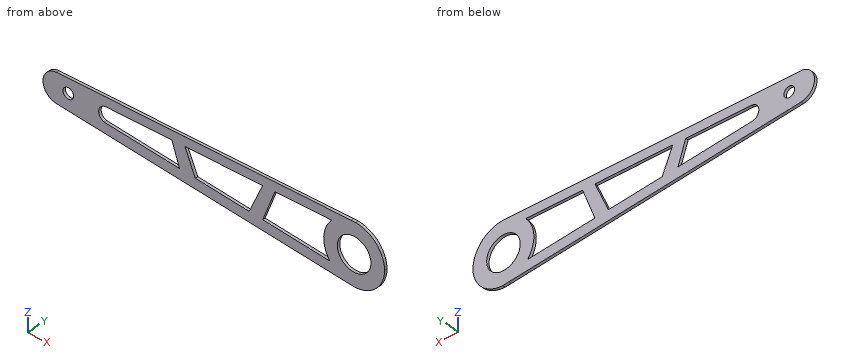
from build123d import *

# Parameters (mm, degrees)
F1_DEPTH = 0.739
F2_R     = 4.5593
F3_DEPTH = 25.4
F4_R     = 1.447766
F5_DEPTH = 25.4


with BuildPart() as f1:
    # F0 (on Front) → F1 (new body)
    with BuildSketch(Plane.XZ):
        with BuildLine():
            ThreePointArc((27.782233, 3.263093), (30.16178, 5.045361), (33.017843, 5.870969))
            Line((33.017843, 5.870969), (-46.981648, 3.796947))
            ThreePointArc((-46.981648, 3.796947), (-50.678208, -0.180343), (-46.9984, -4.173137))
            Line((-46.9984, -4.173137), (32.345508, -10.48937))
            ThreePointArc((32.345508, -10.48937), (29.496427, -9.389113), (27.240975, -7.329802))
            Line((27.240975, -7.329802), (9.005115, -5.878122))
            Line((9.005115, -5.878122), (5.326605, -5.585291))
            Line((5.326605, -5.585291), (-9.280345, -4.422494))
            Line((-9.280345, -4.422494), (-13.580459, -4.08018))
            Line((-13.580459, -4.08018), (-34.080148, -2.448286))
            ThreePointArc((-34.080148, -2.448286), (-35.521395, -0.140366), (-33.488405, 1.668126))
            Line((-33.488405, 1.668126), (-15.681088, 2.131677))
            Line((-15.681088, 2.131677), (-12.137563, 2.223921))
            Line((-12.137563, 2.223921), (9.005115, 2.774297))
            Line((9.005115, 2.774297), (12.333791, 2.860947))
            Line((12.333791, 2.860947), (27.782233, 3.263093))
        make_face()
        with BuildLine():
            ThreePointArc((34.046986, -10.624817), (39.766374, -8.134536), (42.119023, -2.357172))
            ThreePointArc((42.119023, -2.357172), (39.837821, 3.346097), (34.252707, 5.902984))
            Line((34.252707, 5.902984), (33.017843, 5.870969))
            ThreePointArc((33.017843, 5.870969), (30.16178, 5.045361), (27.782233, 3.263093))
            ThreePointArc((27.782233, 3.263093), (25.589768, -1.935156), (27.240975, -7.329802))
            ThreePointArc((27.240975, -7.329802), (29.496427, -9.389113), (32.345508, -10.48937))
            Line((32.345508, -10.48937), (34.046986, -10.624817))
        make_face()
        Polygon((9.005115, -5.878122), (12.333791, 2.860947), (9.005115, 2.774297), (5.326605, -5.585291), align=None)
        Polygon((-9.280345, -4.422494), (-12.137563, 2.223921), (-15.681088, 2.131677), (-13.580459, -4.08018), align=None)
    extrude(amount=F1_DEPTH)

    # F2 (on face) → F3 (cut)
    with BuildSketch(Plane.XZ.offset(0.739)):
        with Locations((33.849008, -2.357172)):
            Circle(F2_R)
    extrude(amount=-F3_DEPTH, mode=Mode.SUBTRACT)

    # F4 (on face) → F5 (cut)
    with BuildSketch(Plane.XZ.offset(0.739)):
        with Locations((-43.807384, 0)):
            Circle(F4_R)
    extrude(amount=-F5_DEPTH, mode=Mode.SUBTRACT)


solid = f1.part
Can you work these out from the model? Positions are in its coordinate system, mm. Coordinates: 2 decimals unless noted, no trailing zeros. Loops run counter-clockwise (first coordinate to the right, second up) from the corner with the lowest first, then second, coordinate; pieces in that order, holes last. Notation, with made-up numbers: (30.25, 8) - (46.25, 8) arc R17 ccw to (46.25, 36) - close; hole circle Ø3 at (64, 51.5). An arc over 180 degrees is marked (long way). Answer as a JSON object with one key per item and string values. Group by question number.
Item 1: If we section it at C-C (x = 6.5): List the corners of the cut face in (y, z) for me, plus the area to 3 significant figures.
Item 2: For pin 1 (8 mm diameter, centred on x = 33.85, z = -2.36, fed in from +Y), with a flat end and sliding along its axis, tell me the tip position at first contact or that it passes through.
Item 3: If we section it at D-D (x = 31.5): List the corners of the cut face in (y, z) for me.
Item 4: If we section it at B-B (z = 0): List the corners of the cut face in (x, y) for me.
Item 5: If I drill on L1, parallel to Z at x = 27, y = -0.25; L2, parallel to Z at x = 34, y = -0.3; L3, parallel to X at y = -0.35, z = -1.5, over which ranges is the centre line in solid material (lowest first)? Write a range as from..to.
Item 6: If we section it at A-A (y = -0.6): List the corners of the cut face in (x, z) for me, plus the area to 3 significant figures.
Returned:
{
 "1": {"outline": "(-0.74, -8.43) - (0, -8.43) - (0, -2.92) - (-0.74, -2.92) - close; (-0.74, 2.71) - (0, 2.71) - (0, 5.18) - (-0.74, 5.18) - close", "area": "5.90 mm²"},
 "2": {"pin 1": "passes through"},
 "3": {"outline": "(-0.74, -10.42) - (0, -10.42) - (0, -6.26) - (-0.74, -6.26) - close; (-0.74, 1.55) - (0, 1.55) - (0, 5.83) - (-0.74, 5.83) - close"},
 "4": {"outline": "(-50.67, -0.74) - (-45.26, -0.74) - (-45.26, 0) - (-50.67, 0) - close; (-42.36, -0.74) - (-35.5, -0.74) - (-35.5, 0) - (-42.36, 0) - close; (-14.96, -0.74) - (-11.18, -0.74) - (-11.18, 0) - (-14.96, 0) - close; (7.78, -0.74) - (11.24, -0.74) - (11.24, 0) - (7.78, 0) - close; (25.92, -0.74) - (29.95, -0.74) - (29.95, 0) - (25.92, 0) - close; (37.75, -0.74) - (41.78, -0.74) - (41.78, 0) - (37.75, 0) - close"},
 "5": {"L1": "z = -10.06..-7.31, -6.99..2.28, 3.24..5.71", "L2": "z = -10.62..-6.91, 2.2..5.9", "L3": "x = -50.46..-35.26, -14.45..-10.54, 7.12..10.67, 25.62..29.37, 38.33..42.07"},
 "6": {"outline": "(-47, -4.17) - (32.35, -10.49) - (34.05, -10.62) arc R8.27 ccw to (42.12, -2.36) arc R8.27 ccw to (34.25, 5.9) - (33.02, 5.87) - (-46.98, 3.8) arc R4 ccw to start; hole circle Ø2.9 at (-43.81, 0); hole (-34.08, -2.45) - (-13.58, -4.08) - (-15.68, 2.13) - (-33.49, 1.67) arc R2.11 ccw to start; hole (-12.14, 2.22) - (-9.28, -4.42) - (5.33, -5.59) - (9.01, 2.77) - close; hole (9.01, -5.88) - (27.24, -7.33) arc R8.27 cw to (27.78, 3.26) - (12.33, 2.86) - close; hole circle Ø9.12 at (33.85, -2.36)", "area": "659 mm²"}
}
